```python
from build123d import *

# Parameters (mm, degrees)
SKETCH1_W                    = 615
SKETCH1_H                    = 105
BASE_FLANGE1_DEPTH           = 1
EDGE_FLANGE1_STRIP_W         = 6
EDGE_FLANGE1_STRIP_H         = 1
EDGE_FLANGE1_STRIP_CUT_DEPTH = 615
EDGE_FLANGE1_DEPTH           = 615
SKETCH16_W                   = 615
SKETCH16_H                   = 196.52545168
CUT_EXTRUDE1_DEPTH           = 10
SWEPT_START                  = -307.5
SWEPT_FLANGE1_DEPTH          = 615
EDGE_FLANGE2_DEPTH           = 84
EDGE_FLANGE2_BEND_DEPTH      = 84
CUT_EXTRUDE2_DEPTH           = 623.622700982
CUT_EXTRUDE2_DEPTH_BACK      = 623.622700982
SKETCH39_R                   = 2.5
FILLET1_R                    = 8
SKETCH45_R                   = 1.5
CUT_EXTRUDE3_DEPTH           = 10


# Read off the part's stored shape, not the designer's step: Swept Flange1
# Sheet-metal steps are written as plain solids
with BuildPart() as part:
    # Sketch1 → Base-Flange1 (new body)
    with BuildSketch(Plane(origin=(0, 0, 0), x_dir=(1, 0, 0), z_dir=(0, 1, 0))):
        Rectangle(SKETCH1_W, SKETCH1_H)
    extrude(amount=-BASE_FLANGE1_DEPTH)

    # Edge-Flange1 strip (across the edge) → Edge-Flange1 strip cut (cut)
    with BuildSketch(Plane(origin=(307.5, -1, 52.5), x_dir=(0, 0, -1), z_dir=(-1, 0, 0))):
        with Locations((-2, -0.5)):
            Rectangle(EDGE_FLANGE1_STRIP_W, EDGE_FLANGE1_STRIP_H)
    extrude(amount=EDGE_FLANGE1_STRIP_CUT_DEPTH, mode=Mode.SUBTRACT)

    # Edge-Flange1 section (across the edge) → Edge-Flange1 (add)
    with BuildSketch(Plane(origin=(307.5, -1, 52.5), x_dir=(0, 0, -1), z_dir=(-1, 0, 0))):
        with BuildLine():
            Line((-1, 1), (-1, 7))
            Line((-1, 7), (0, 7))
            Line((0, 7), (0, 1))
            ThreePointArc((0, 1), (0.292893219, 0.292893219), (1, 0))
            Line((1, 0), (1, -1))
            ThreePointArc((1, -1), (-0.414213562, -0.414213562), (-1, 1))
        make_face()
    extrude(amount=EDGE_FLANGE1_DEPTH)

    # Sketch16 → Cut-Extrude1 (cut)
    with BuildSketch(Plane(origin=(0, 0, 0), x_dir=(1, 0, 0), z_dir=(0, 1, 0))):
        with Locations((0, 130.76272584)):
            Rectangle(SKETCH16_W, SKETCH16_H)
    extrude(amount=-CUT_EXTRUDE1_DEPTH, mode=Mode.SUBTRACT)

    # Swept Flange1 outline → Swept Flange1 (add)
    with BuildSketch(Plane.YZ.offset(SWEPT_START)):
        with BuildLine():
            Line((-1, -51.166666667), (-1, -53.833333333))
            Line((-1, -53.833333333), (0, -53.833333333))
            Line((0, -53.833333333), (0, -51.166666667))
            ThreePointArc((0, -51.166666667), (-0.205266808, -49.901755603), (-0.8, -48.766666667))
            Line((-0.8, -48.766666667), (-4.65, -43.633333333))
            ThreePointArc((-4.65, -43.633333333), (-5.25, -41.833333333), (-4.65, -40.033333333))
            Line((-4.65, -40.033333333), (-0.8, -34.9))
            ThreePointArc((-0.8, -34.9), (-0.205266808, -33.764911064), (0, -32.5))
            Line((0, -32.5), (-1, -32.5))
            ThreePointArc((-1, -32.5), (-1.153950106, -33.448683298), (-1.6, -34.3))
            Line((-1.6, -34.3), (-5.45, -39.433333333))
            ThreePointArc((-5.45, -39.433333333), (-6.25, -41.833333333), (-5.45, -44.233333333))
            Line((-5.45, -44.233333333), (-1.6, -49.366666667))
            ThreePointArc((-1.6, -49.366666667), (-1.153950106, -50.217983369), (-1, -51.166666667))
        make_face()
    extrude(amount=SWEPT_FLANGE1_DEPTH)

    # Edge-Flange2 section (across the edge) → Edge-Flange2 (add)
    with BuildSketch(Plane(origin=(308.5, -1, -32.5), x_dir=(-1, 0, 0), z_dir=(0, 0, 1))):
        with BuildLine():
            Line((-1, 1), (-1, 39))
            Line((-1, 39), (0, 39))
            Line((0, 39), (0, 1))
            ThreePointArc((0, 1), (0.292893219, 0.292893219), (1, 0))
            Line((1, 0), (1, -1))
            ThreePointArc((1, -1), (-0.414213562, -0.414213562), (-1, 1))
        make_face()
    extrude(amount=EDGE_FLANGE2_DEPTH)

    # Edge-Flange2 section 2 (across the edge) → Edge-Flange2 bend (add)
    with BuildSketch(Plane(origin=(-308.5, -1, 51.5), x_dir=(1, 0, 0), z_dir=(0, 0, -1))):
        with BuildLine():
            Line((-1, 1), (-1, 39))
            Line((-1, 39), (0, 39))
            Line((0, 39), (0, 1))
            ThreePointArc((0, 1), (0.292893219, 0.292893219), (1, 0))
            Line((1, 0), (1, -1))
            ThreePointArc((1, -1), (-0.414213562, -0.414213562), (-1, 1))
        make_face()
    extrude(amount=EDGE_FLANGE2_BEND_DEPTH)

    # Sketch39 → Cut-Extrude2 (cut, two sides: drawn at the far end of the back side and taken through both)
    with BuildSketch(Plane.ZY.offset(309.5).offset(-CUT_EXTRUDE2_DEPTH_BACK)):
        with Locations(Location((40, -32.5, 0), (0, 0, 90))):
            Circle(SKETCH39_R)
        with BuildLine():
            Line((-32.5, -10), (19.901558991, -10))
            Line((19.901558991, -10), (34.712752069, -36.876753821))
            ThreePointArc((34.712752069, -36.876753821), (36.929590525, -39.160869046), (40, -40))
            ThreePointArc((40, -40), (43.667304301, -38.758423068), (45.82614719, -35.544386433))
            Line((45.82614719, -35.544386433), (51.5, -14.63988364))
            Line((51.5, -14.63988364), (60.41713226, -14.63988364))
            Line((60.41713226, -14.63988364), (60.41713226, -59.649041705))
            Line((60.41713226, -59.649041705), (-51.871278106, -59.649041705))
            Line((-51.871278106, -59.649041705), (-51.871278106, -10))
            Line((-51.871278106, -10), (-32.5, -10))
        make_face()
    extrude(amount=CUT_EXTRUDE2_DEPTH + CUT_EXTRUDE2_DEPTH_BACK, mode=Mode.SUBTRACT)

    # Fillet1
    fillet1_edges = [part.edges().sort_by_distance(p)[0] for p in [
        (-309, -10, -32.5),
        (309, -10, -32.5),
    ]]
    fillet(fillet1_edges, radius=FILLET1_R)

    # Sketch45 → Cut-Extrude3 (cut)
    with BuildSketch(Plane(origin=(0, -23.92, -17.94), x_dir=(1, 0, 0), z_dir=(0, 0.7999999999999998, 0.6000000000000002))):
        with Locations(Location((0, 35.325, 0), (0, 0, 270))):
            Circle(SKETCH45_R)
    extrude(amount=-CUT_EXTRUDE3_DEPTH, mode=Mode.SUBTRACT)


solid = part.part
```
Geometry check sheet. Reference: the model listing, model coordinates, mm. A direction names the side the tool comes from. Coordinates: 2 decimals unless noted, no trailing zeros. Loops run counter-clockwise (first coordinate to the right, second up) from the corner with the lowest first, then second, coordinate; pieces in that order, holes last. Notation, with made-up numbers: (-10, -33) - (14, -33) arc R12 cw to (14, -18) - close; hole circle Ø11 at (1, -33). An arc over 180 degrees is marked (long way). One line per item, written item: value. Start each with the question number.
(1) Cross-section at C-C on y = -23.5. Enter the section's corners in (x, z).
(2) Cross-section at A-A on x = -96.5. Enter the section's corners in (y, z), plus the area to 3 significant figures.
(3) Material ranges on line 1 (X direction, y = -7, z = 0.5); line 2 (Z direction, x = 260.5, y = -4.5); line 3 (Z direction, x = 170, y = -7.5), recorded low to high. Write a range as [from, to].
(4) Depth check by flat-ended pin: P1, Ø1, axis at x = -309, y = -6, coming from the +Z side; P2, Ø4, axis at x = 162, z = 24, coming from the -Y side; P3, Ø0.6, axis at y = -2.5, z = 52.5, coming from the -X side. Enter the tip coordinate at first touch or a pass-through.
(5) Mould release check, pull along X, two halves, no side actions. Record for faces 4 (the flat face through (-4, 0, 9)), 5 (the flat face through (-308.5, -9, 19)), 6 (the flat face through (-309.5, -12, 29)): released by +X, released by -X, zero draft, split by the parting line, or undercut.
(6) Cross-section at B-B on z = -11.5. Enter the section's corners in (x, y), plus the area to 3 significant figures.
(7) Tool access check on faces 1 (the flat face through (-4, -1, 9)), 2 (the flat face through (308.5, -13, 28)), 3 (the flat face through (309.5, -12, 28)). Record the directions out of +Z, -Z, +X, -X, +Y, -Y that give a thin tool (end or side, any length) a straight path to the whole face; none if there is none.
Results below:
1. outline: (-309.5, 27.34) - (-308.5, 27.34) - (-308.5, 49.1) - (-309.5, 49.1) - close; (308.5, 27.34) - (309.5, 27.34) - (309.5, 49.1) - (308.5, 49.1) - close
2. outline: (-8, 52.5) - (-2, 52.5) arc R1 cw to (-1, 51.5) - (-1, -32.5) arc R3 cw to (-1.6, -34.3) - (-5.45, -39.43) arc R4 ccw to (-5.45, -44.23) - (-1.6, -49.37) arc R3 cw to (-1, -51.17) - (-1, -53.83) - (0, -53.83) - (0, -51.17) arc R4 ccw to (-0.8, -48.77) - (-4.65, -43.63) arc R3 cw to (-4.65, -40.03) - (-0.8, -34.9) arc R4 ccw to (0, -32.5) - (0, 51.5) arc R2 ccw to (-2, 53.5) - (-8, 53.5) - close
2. area: 117 mm2
3. line 1: x = [-309.5, -308.5], [308.5, 309.5]
3. line 2: z = [-45.5, -43.83], [-39.83, -38.17], [52.5, 53.5]
3. line 3: z = [52.5, 53.5]
4. P1: stops at z = 51.5
4. P2: stops at y = -1
4. P3: stops at x = -307.5
5. face 4: zero draft
5. face 5: undercut
5. face 6: released by -X
6. outline: (-309.5, -10) - (-308.5, -10) - (-308.5, -2) arc R1 cw to (-307.5, -1) - (307.5, -1) arc R1 cw to (308.5, -2) - (308.5, -10) - (309.5, -10) - (309.5, -2) arc R2 ccw to (307.5, 0) - (-307.5, 0) arc R2 ccw to (-309.5, -2) - close
6. area: 636 mm2
7. face 1: -Y
7. face 2: +Z, -Z, -Y
7. face 3: +Z, -Z, +X, +Y, -Y
